The model under review builds one solid part; all positions refer to its coordinate system, in mm. A direction names the side the tool comes from. Round coordinates to 2 decimals unless told otherwise and drop trailing zeros. Write each loop counter-clockwise with the first axis right and the second up, starting at its lowest first coordinate (ties: lowest second). Pieces come first, ordered by that corner, then holes. Notation, with made-up numbers: (80, -6) - (130, -6) arc R14 ccw to (130, 17) - close; hole circle Ø1 at (56, 2.5). An arc over 180 degrees is marked (long way). Write each question's results on one line, items separated by ' | '.
```python
from build123d import *

# Parameters (mm, degrees)
F0_W     = 15.83
F0_H     = 15.83
F0_R     = 2.435
F1_DEPTH = 9.53
F2_DEPTH = 1.77
F3_W     = 13.17
F3_H     = 13.5795233832
F3_R     = 4.0052383084
F3_R_2   = 3.0452383084
F4_DEPTH = 8.54


with BuildPart() as f1:
    # F0 (on Top) → F1 (new body)
    with BuildSketch(Plane.XY):
        with Locations((-0.0172966565, -0.2047616916)):
            Rectangle(F0_W, F0_H)
        with Locations((-4.0272966565, -4.2147616916)):
            Circle(F0_R, mode=Mode.SUBTRACT)
        with Locations((3.9926922612, -4.2280943334)):
            Circle(F0_R, mode=Mode.SUBTRACT)
        with Locations((-4.0272966565, 3.8052383084)):
            Circle(F0_R, mode=Mode.SUBTRACT)
        with Locations((3.9927033435, 3.8052383084)):
            Circle(F0_R, mode=Mode.SUBTRACT)
        with Locations((-4.0272966565, -4.2147616916)):
            Circle(F0_R)
        with Locations((3.9926922612, -4.2280943334)):
            Circle(F0_R)
        with Locations((3.9927033435, 3.8052383084)):
            Circle(F0_R)
        with Locations((-4.0272966565, 3.8052383084)):
            Circle(F0_R)
    extrude(amount=F1_DEPTH)

    # F0 (on Top) → F2 (join)
    with BuildSketch(Plane.XY):
        with Locations((-4.0272966565, -4.2147616916)):
            Circle(F0_R)
        with Locations((3.9926922612, -4.2280943334)):
            Circle(F0_R)
        with Locations((-4.0272966565, 3.8052383084)):
            Circle(F0_R)
        with Locations((3.9927033435, 3.8052383084)):
            Circle(F0_R)
    extrude(amount=-F2_DEPTH)

    # F3 (on face) → F4 (cut)
    with BuildSketch(Plane.XY.offset(9.53)):
        with Locations((-0.0172966565, 0)):
            Rectangle(F3_W, F3_H)
        with Locations((-0.2220583481, 0)):
            Circle(F3_R, mode=Mode.SUBTRACT)
        with Locations((-0.2220583481, 0)):
            Circle(F3_R_2)
    extrude(amount=-F4_DEPTH, mode=Mode.SUBTRACT)


solid = f1.part
```
Q1. We need section D-D (y = 0). State the section outline as (x, z) points, plus the area to 3 significant figures.
Evaluation:
outline: (-7.93, 0) - (7.9, 0) - (7.9, 9.53) - (6.57, 9.53) - (6.57, 0.99) - (3.78, 0.99) - (3.78, 9.53) - (2.82, 9.53) - (2.82, 0.99) - (-3.27, 0.99) - (-3.27, 9.53) - (-4.23, 9.53) - (-4.23, 0.99) - (-6.6, 0.99) - (-6.6, 9.53) - (-7.93, 9.53) - close | area: 54.8 mm^2
Q2. We need section B-B (y = 6.5). State the section outline as (x, z) points, plus the area to 3 significant figures.
Evaluation:
outline: (-7.93, 0) - (7.9, 0) - (7.9, 9.53) - (6.57, 9.53) - (6.57, 0.99) - (-6.6, 0.99) - (-6.6, 9.53) - (-7.93, 9.53) - close | area: 38.4 mm^2
Q3. Tool access review of faces 4 (the cylindrical face through (2.2, -2.58, -0.87)), 5 (the flat face through (1, 3, 9.53)), 6 (the flat face through (-6.602, 0, 5)): name each direction out of +Z, -Z, +X, -X, +Y, -Y from which nothing blocks a thin tool from reaching the whole face with its end or side.
Evaluation:
face 4: -Z | face 5: +Z, +X, -X, +Y, -Y | face 6: +Z
Q4. We need section A-A (z = 3.75). State the section outline as (x, y) points.
Evaluation:
outline: (-7.93, -8.12) - (7.9, -8.12) - (7.9, 7.71) - (-7.93, 7.71) - close; circle Ø8.01 at (-0.22, 0); hole (-6.6, -6.79) - (6.57, -6.79) - (6.57, 6.79) - (-6.6, 6.79) - close; hole circle Ø6.09 at (-0.22, 0)
Q5. We need section C-C (x = 2). State the section outline as (y, z) points, plus the area to 3 significant figures.
Evaluation:
outline: (-8.12, 0) - (-5.63, 0) - (-5.63, -1.77) - (-2.83, -1.77) - (-2.83, 0) - (2.41, 0) - (2.41, -1.77) - (5.2, -1.77) - (5.2, 0) - (7.71, 0) - (7.71, 9.53) - (6.79, 9.53) - (6.79, 0.99) - (3.33, 0.99) - (3.33, 9.53) - (2.08, 9.53) - (2.08, 0.99) - (-2.08, 0.99) - (-2.08, 9.53) - (-3.33, 9.53) - (-3.33, 0.99) - (-6.79, 0.99) - (-6.79, 9.53) - (-8.12, 9.53) - close | area: 66.1 mm^2
Q6. Insertion check: P1, Ø6, axis at x = 5, y = -6, coming from the +Z side; P2, Ø2, axis at x = 5, y = 3.5, coming from the +Z side; P3, Ø1, axis at x = -3.5, y = -0.5, coming from the -Z side. Each pin has a flat end and moves straight along its axis. Give the tip position at first contact, or say it passes through.
Evaluation:
P1: stops at z = 9.53 | P2: stops at z = 0.99 | P3: stops at z = 0
Q7. The part is to be moulded in two halves that separate along X. For faces 1 (the flat face through (-4, -4, -1.77)), 2 (the flat face through (7.898, 0, 5)), 3 (the flat face through (6.568, 0, 5)), say which applies: released by +X, released by -X, zero draft, split by the parting line, or undercut.
Evaluation:
face 1: zero draft | face 2: released by +X | face 3: undercut
Q8. For probe 1 along X at (y, z) = (4.5, 2.5); probe 2 along Y at (x, z) = (5, 1.25); probe 3 along Y at (x, z) = (3, 8.75), list the stretches that pass through material, from the lowest coordinate up.
Evaluation:
probe 1: x = -7.93 to -6.6, 6.57 to 7.9 | probe 2: y = -8.12 to -6.79, 6.79 to 7.71 | probe 3: y = -8.12 to -6.79, -2.38 to 2.38, 6.79 to 7.71
